Verification items for the finished model (mm, model axes). Round coordinates to 2 decimals unless told otherwise and drop trailing zeros. Loops run counter-clockwise (first coordinate to the right, second up) from the corner with the lowest first, then second, coordinate; pieces in that order, holes last. Notation, with made-up numbers: M 34,-28.75 L 73,-28.75 A18 ccw 73,-7.75 Z; hole C 69,-31 d10. An arc over 180 degrees is marked long. Write item = value, one per line. Start each with the question number.
from build123d import *

# Parameters (mm, degrees)
SKETCH1_R           = 3.225
BOSS_EXTRUDE1_DEPTH = 0.8


with BuildPart() as part:
    # Sketch1 → Boss-Extrude1 (new body)
    with BuildSketch(Plane.XY):
        with BuildLine():
            ThreePointArc((4.65, 25.4), (0, 30.05), (-4.65, 25.4))
            Line((-4.65, 25.4), (-4.65, 23))
            ThreePointArc((-4.65, 23), (-5.235786438, 21.585786438), (-6.65, 21))
            Line((-6.65, 21), (-8.759132098, 21))
            Line((-8.759132098, 21), (-21, 21))
            Line((-21, 21), (-21, 7.133487824))
            Line((-21, 7.133487824), (-21, 6.65))
            ThreePointArc((-21, 6.65), (-21.585786438, 5.235786438), (-23, 4.65))
            Line((-23, 4.65), (-25.4, 4.65))
            ThreePointArc((-25.4, 4.65), (-30.05, 0), (-25.4, -4.65))
            Line((-25.4, -4.65), (-23, -4.65))
            ThreePointArc((-23, -4.65), (-21.585786438, -5.235786438), (-21, -6.65))
            Line((-21, -6.65), (-21, -8.759132098))
            Line((-21, -8.759132098), (-21, -21))
            Line((-21, -21), (-7.133487824, -21))
            Line((-7.133487824, -21), (-6.65, -21))
            ThreePointArc((-6.65, -21), (-5.235786438, -21.585786438), (-4.65, -23))
            Line((-4.65, -23), (-4.65, -25.4))
            ThreePointArc((-4.65, -25.4), (0, -30.05), (4.65, -25.4))
            Line((4.65, -25.4), (4.65, -23))
            ThreePointArc((4.65, -23), (5.235786438, -21.585786438), (6.65, -21))
            Line((6.65, -21), (8.759132098, -21))
            Line((8.759132098, -21), (21, -21))
            Line((21, -21), (21, -7.133487824))
            Line((21, -7.133487824), (21, -6.65))
            ThreePointArc((21, -6.65), (21.585786438, -5.235786438), (23, -4.65))
            Line((23, -4.65), (25.4, -4.65))
            ThreePointArc((25.4, -4.65), (30.05, 0), (25.4, 4.65))
            Line((25.4, 4.65), (23, 4.65))
            ThreePointArc((23, 4.65), (21.585786438, 5.235786438), (21, 6.65))
            Line((21, 6.65), (21, 8.759132098))
            Line((21, 8.759132098), (21, 21))
            Line((21, 21), (7.133487824, 21))
            Line((7.133487824, 21), (6.65, 21))
            ThreePointArc((6.65, 21), (5.235786438, 21.585786438), (4.65, 23))
            Line((4.65, 23), (4.65, 25.4))
        make_face()
        with Locations((0, -25.4)):
            Circle(SKETCH1_R, mode=Mode.SUBTRACT)
        with Locations((25.4, 0)):
            Circle(SKETCH1_R, mode=Mode.SUBTRACT)
        with Locations((-25.4, 0)):
            Circle(SKETCH1_R, mode=Mode.SUBTRACT)
        with Locations((0, 25.4)):
            Circle(SKETCH1_R, mode=Mode.SUBTRACT)
    extrude(amount=BOSS_EXTRUDE1_DEPTH)


solid = part.part
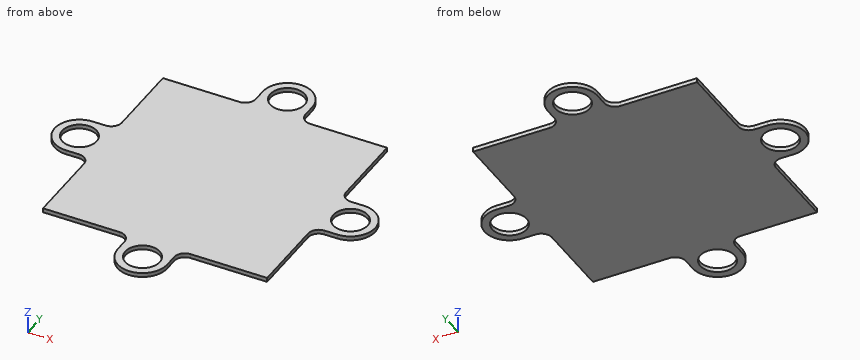
1. Gauge pin test, flat ends, axial feed: P1, Ø5, axis at x = 0, y = 25.4, coming from the +Z side; P2, Ø1, axis at x = 17, y = -18.5, coming from the -Z side. Record the tip position at first contact, or that the pin passes through.
2. Thickness scan on line 1 (Y direction, x = 0, z = 0.4) (3 decimals); line 2 (Y direction, x = 25.4, z = 0.3) (3 decimals); line 3 (X direction, y = 26, z = 0.15). Record the ranges inside material, lowest first.
3. Section check A-A, the plane x = 0. Enter the section's corners in (y, z) (3 decimals), and give its area (3 significant figures).
4. Section check D-D, the plane y = -13. Enter the section's corners in (x, z), and give its area (3 significant figures).
5. Section check C-C, the plane z = 0.4. Give the number of separate pieces and of enclosed holes in the cut face, and give its area (3 significant figures).
Computed values:
q1.P1 = through
q1.P2 = 0
q2.line_1 = -30.05 to -28.625, -22.175 to 22.175, 28.625 to 30.05
q2.line_2 = -4.65 to -3.225, 3.225 to 4.65
q2.line_3 = -4.61 to -3.17, 3.17 to 4.61
q3.outline = M -30.05,0 L -28.625,0 L -28.625,0.8 L -30.05,0.8 Z; M -22.175,0 L 22.175,0 L 22.175,0.8 L -22.175,0.8 Z; M 28.625,0 L 30.05,0 L 30.05,0.8 L 28.625,0.8 Z
q3.area = 37.8 mm2
q4.outline = M -21,0 L 21,0 L 21,0.8 L -21,0.8 Z
q4.area = 33.6 mm2
q5.separate_pieces = 1
q5.enclosed_holes = 4
q5.area = 1,940 mm2
